Could you check a few things on this model? Use its own coordinates, in mm. A direction names the side the tool comes from. Coordinates: 2 decimals unless noted, no trailing zeros. Loops run counter-clockwise (first coordinate to the right, second up) from the corner with the lowest first, then second, coordinate; pieces in that order, holes last. Notation, with made-up numbers: (-8, 46) - (45, 46) arc R20 cw to (45, 60) - close; hole circle Ø5 at (44.25, 29). An arc over 180 degrees is marked (long way). Use CSV: the item, a comma, the result in double quotes.
Autodesk Fusion 360 part; units mm, degrees
sketch "Sketch1" plane through (0, 0, 0) normal (0, 0, 1) x (1, 0, 0)
  arc A0 (-0.5916, 85.05) -> (-0.493, 85.1333) centre (-0.5916, 85.15) ccw
  line L0 (-0.5916, 85.05) -> (-0.9084, 85.05)
  arc A1 (-1.007, 85.1333) -> (-1.5833, 84.557) centre (-1.5, 85.05) ccw
  arc A2 (0.0833, 84.557) -> (-0.493, 85.1333) centre (0, 85.05) ccw
  arc A3 (-1.007, 85.1333) -> (-0.9084, 85.05) centre (-0.9084, 85.15) ccw
  arc A4 (-1.5, 84.4584) -> (-1.5833, 84.557) centre (-1.6, 84.4584) ccw
  line L1 (-1.5, 84.4584) -> (-1.5, 0.5916)
  line L2 (0, 0.5916) -> (0, 84.4584)
  arc A5 (0.0833, 84.557) -> (0, 84.4584) centre (0.1, 84.4584) ccw
  line L3 (-1.5, 42.525) -> (0, 42.525) construction
  arc A6 (0, 0.5916) -> (0.0833, 0.493) centre (0.1, 0.5916) ccw
  arc A7 (-1.5833, 0.493) -> (-1.5, 0.5916) centre (-1.6, 0.5916) ccw
  arc A8 (-0.9084, 0) -> (-1.007, -0.0833) centre (-0.9084, -0.1) ccw
  arc A9 (-1.5833, 0.493) -> (-1.007, -0.0833) centre (-1.5, 0) ccw
  line L4 (-0.5916, 0) -> (-0.9084, 0)
  arc A10 (-0.493, -0.0833) -> (-0.5916, 0) centre (-0.5916, -0.1) ccw
  arc A11 (-0.493, -0.0833) -> (0.0833, 0.493) centre (0, 0) ccw
  line L5 (-3.5, 87.05) -> (12.65, 87.05)
  line L6 (12.65, 87.05) -> (12.65, -2)
  line L7 (12.65, -2) -> (-3.5, -2)
  line L8 (-3.5, -2) -> (-3.5, 87.05)
  line L9 (2.9334, 0) -> (2.5916, 0)
  line L10 (2, 84.4584) -> (2, 0.5916)
  arc A12 (3.6083, 84.557) -> (3.525, 84.4584) centre (3.625, 84.4584) ccw
  arc A13 (2.9334, 85.05) -> (3.032, 85.1333) centre (2.9334, 85.15) ccw
  arc A14 (1.9167, 0.493) -> (2.493, -0.0833) centre (2, 0) ccw
  arc A15 (2.493, 85.1333) -> (2.5916, 85.05) centre (2.5916, 85.15) ccw
  arc A16 (3.032, -0.0833) -> (3.6083, 0.493) centre (3.525, 0) ccw
  arc A17 (2, 84.4584) -> (1.9167, 84.557) centre (1.9, 84.4584) ccw
  arc A18 (3.525, 0.5916) -> (3.6083, 0.493) centre (3.625, 0.5916) ccw
  line L11 (2.9334, 85.05) -> (2.5916, 85.05)
  arc A19 (2.5916, 0) -> (2.493, -0.0833) centre (2.5916, -0.1) ccw
  line L12 (2, 42.525) -> (3.525, 42.525) construction
  arc A20 (2.493, 85.1333) -> (1.9167, 84.557) centre (2, 85.05) ccw
  arc A21 (3.6083, 84.557) -> (3.032, 85.1333) centre (3.525, 85.05) ccw
  arc A22 (3.032, -0.0833) -> (2.9334, 0) centre (2.9334, -0.1) ccw
  arc A23 (1.9167, 0.493) -> (2, 0.5916) centre (1.9, 0.5916) ccw
  line L13 (3.525, 0.5916) -> (3.525, 84.4584)
  arc A24 (5.4417, 0.493) -> (6.018, -0.0833) centre (5.525, 0) ccw
  line L14 (10.65, 0.5916) -> (10.65, 84.4584)
  line L15 (7.075, 0.5916) -> (7.075, 84.4584)
  line L16 (9.075, 42.525) -> (10.65, 42.525) construction
  arc A25 (9.568, 85.1333) -> (8.9917, 84.557) centre (9.075, 85.05) ccw
  line L17 (5.525, 84.4584) -> (5.525, 0.5916)
  arc A26 (6.582, -0.0833) -> (7.1583, 0.493) centre (7.075, 0) ccw
  arc A27 (10.157, -0.0833) -> (10.7333, 0.493) centre (10.65, 0) ccw
  arc A28 (6.018, 85.1333) -> (5.4417, 84.557) centre (5.525, 85.05) ccw
  line L18 (10.0584, 85.05) -> (9.6666, 85.05)
  arc A29 (8.9917, 0.493) -> (9.075, 0.5916) centre (8.975, 0.5916) ccw
  line L19 (6.4834, 0) -> (6.1166, 0)
  arc A30 (6.018, 85.1333) -> (6.1166, 85.05) centre (6.1166, 85.15) ccw
  arc A31 (9.568, 85.1333) -> (9.6666, 85.05) centre (9.6666, 85.15) ccw
  arc A32 (7.075, 0.5916) -> (7.1583, 0.493) centre (7.175, 0.5916) ccw
  line L20 (5.525, 42.525) -> (7.075, 42.525) construction
  arc A33 (6.1166, 0) -> (6.018, -0.0833) centre (6.1166, -0.1) ccw
  arc A34 (7.1583, 84.557) -> (7.075, 84.4584) centre (7.175, 84.4584) ccw
  line L21 (6.4834, 85.05) -> (6.1166, 85.05)
  arc A35 (9.075, 84.4584) -> (8.9917, 84.557) centre (8.975, 84.4584) ccw
  line L22 (9.075, 84.4584) -> (9.075, 0.5916)
  arc A36 (10.7333, 84.557) -> (10.65, 84.4584) centre (10.75, 84.4584) ccw
  arc A37 (6.582, -0.0833) -> (6.4834, 0) centre (6.4834, -0.1) ccw
  arc A38 (8.9917, 0.493) -> (9.568, -0.0833) centre (9.075, 0) ccw
  arc A39 (6.4834, 85.05) -> (6.582, 85.1333) centre (6.4834, 85.15) ccw
  arc A40 (7.1583, 84.557) -> (6.582, 85.1333) centre (7.075, 85.05) ccw
  arc A41 (9.6666, 0) -> (9.568, -0.0833) centre (9.6666, -0.1) ccw
  arc A42 (10.7333, 84.557) -> (10.157, 85.1333) centre (10.65, 85.05) ccw
  line L23 (10.0584, 0) -> (9.6666, 0)
  arc A43 (5.525, 84.4584) -> (5.4417, 84.557) centre (5.425, 84.4584) ccw
  arc A44 (10.65, 0.5916) -> (10.7333, 0.493) centre (10.75, 0.5916) ccw
  arc A45 (10.157, -0.0833) -> (10.0584, 0) centre (10.0584, -0.1) ccw
  arc A46 (5.4417, 0.493) -> (5.525, 0.5916) centre (5.425, 0.5916) ccw
  arc A47 (10.0584, 85.05) -> (10.157, 85.1333) centre (10.0584, 85.15) ccw
  arc A48 (9.568, 85.1333) -> (9.6666, 85.05) centre (9.6666, 85.15) ccw
  arc A49 (6.4834, 85.05) -> (6.582, 85.1333) centre (6.4834, 85.15) ccw
  arc A50 (10.0584, 85.05) -> (10.157, 85.1333) centre (10.0584, 85.15) ccw
  arc A51 (6.018, 85.1333) -> (5.4417, 84.557) centre (5.525, 85.05) ccw
  line L24 (10.0584, 85.05) -> (9.6666, 85.05)
  arc A52 (2.9334, 85.05) -> (3.032, 85.1333) centre (2.9334, 85.15) ccw
  arc A53 (10.7333, 84.557) -> (10.157, 85.1333) centre (10.65, 85.05) ccw
  arc A54 (6.018, 85.1333) -> (6.1166, 85.05) centre (6.1166, 85.15) ccw
  arc A55 (5.525, 84.4584) -> (5.4417, 84.557) centre (5.425, 84.4584) ccw
  arc A56 (2, 84.4584) -> (1.9167, 84.557) centre (1.9, 84.4584) ccw
  arc A57 (0.0833, 84.557) -> (0, 84.4584) centre (0.1, 84.4584) ccw
  arc A58 (10.7333, 84.557) -> (10.65, 84.4584) centre (10.75, 84.4584) ccw
  arc A59 (-1.007, 85.1333) -> (-1.5833, 84.557) centre (-1.5, 85.05) ccw
  line L25 (2.9334, 85.05) -> (2.5916, 85.05)
  arc A60 (3.6083, 84.557) -> (3.032, 85.1333) centre (3.525, 85.05) ccw
  arc A61 (-1.007, 85.1333) -> (-0.9084, 85.05) centre (-0.9084, 85.15) ccw
  arc A62 (7.1583, 84.557) -> (6.582, 85.1333) centre (7.075, 85.05) ccw
  arc A63 (2.493, 85.1333) -> (1.9167, 84.557) centre (2, 85.05) ccw
  arc A64 (9.075, 84.4584) -> (8.9917, 84.557) centre (8.975, 84.4584) ccw
  line L26 (-0.5916, 85.05) -> (-0.9084, 85.05)
  arc A65 (0.0833, 84.557) -> (-0.493, 85.1333) centre (0, 85.05) ccw
  arc A66 (-1.5, 84.4584) -> (-1.5833, 84.557) centre (-1.6, 84.4584) ccw
  arc A67 (-0.5916, 85.05) -> (-0.493, 85.1333) centre (-0.5916, 85.15) ccw
  arc A68 (7.1583, 84.557) -> (7.075, 84.4584) centre (7.175, 84.4584) ccw
  arc A69 (2.493, 85.1333) -> (2.5916, 85.05) centre (2.5916, 85.15) ccw
  line L27 (6.4834, 85.05) -> (6.1166, 85.05)
  arc A70 (3.6083, 84.557) -> (3.525, 84.4584) centre (3.625, 84.4584) ccw
  arc A71 (9.568, 85.1333) -> (8.9917, 84.557) centre (9.075, 85.05) ccw
  point P0 (-3.5, 87.05)
  point P1 (3.525, 0)
  point P2 (0.5, 87.05)
  point P3 (10.65, 0)
  point P4 (6.3, 0)
  dimension "d1" = 0.5
  dimension "d2" = 0.1
  dimension "d3" = 1.5
  dimension "d10" = 85.05
  dimension "d12" = 2
  dimension "d13" = 2
  dimension "d14" = 2
  dimension "d15" = 0.5
  dimension "d16" = 0.1
  dimension "d17" = 1.525
  dimension "d20" = 0.5
  dimension "d21" = 0.1
  dimension "d22" = 1.55
  dimension "d24" = 0.5
  dimension "d25" = 0.1
  dimension "d26" = 1.575
  dimension "d29" = 2
  dimension "d30" = 2
  dimension "d32" = 2
  dimension "d38" = 0.5
  dimension "d39" = 0.1
  dimension "d40" = 0.5
  dimension "d41" = 0.1
  dimension "d42" = 0.5
  dimension "d43" = 0.1
  dimension "d44" = 0.5
  dimension "d45" = 0.1
  dimension "d46" = 2
extrude "Extrude1" add sketch "Sketch1" along normal blind 14
sketch "Sketch2" plane through (0, 0, 0) normal (0, 0, -1) x (1, 0, 0)
  arc A0 (6.582, -85.1333) -> (7.1583, -84.557) centre (7.075, -85.05) ccw
  arc A1 (6.582, -85.1333) -> (6.4834, -85.05) centre (6.4834, -85.15) ccw
  line L0 (6.4834, -85.05) -> (6.1166, -85.05)
  arc A2 (6.1166, -85.05) -> (6.018, -85.1333) centre (6.1166, -85.15) ccw
  arc A3 (5.4417, -84.557) -> (6.018, -85.1333) centre (5.525, -85.05) ccw
  arc A4 (5.4417, -84.557) -> (5.525, -84.4584) centre (5.425, -84.4584) ccw
  line L1 (5.525, -84.4584) -> (5.525, -0.5916)
  arc A5 (5.525, -0.5916) -> (5.4417, -0.493) centre (5.425, -0.5916) ccw
  arc A6 (6.018, 0.0833) -> (5.4417, -0.493) centre (5.525, 0) ccw
  arc A7 (6.018, 0.0833) -> (6.1166, 0) centre (6.1166, 0.1) ccw
  line L2 (6.1166, 0) -> (6.4834, 0)
  arc A8 (6.4834, 0) -> (6.582, 0.0833) centre (6.4834, 0.1) ccw
  arc A9 (7.1583, -0.493) -> (6.582, 0.0833) centre (7.075, 0) ccw
  arc A10 (7.1583, -0.493) -> (7.075, -0.5916) centre (7.175, -0.5916) ccw
  line L3 (7.075, -0.5916) -> (7.075, -84.4584)
  arc A11 (7.075, -84.4584) -> (7.1583, -84.557) centre (7.175, -84.4584) ccw
  line L4 (10.0584, -85.05) -> (9.6666, -85.05)
  arc A12 (9.6666, -85.05) -> (9.568, -85.1333) centre (9.6666, -85.15) ccw
  arc A13 (8.9917, -84.557) -> (9.568, -85.1333) centre (9.075, -85.05) ccw
  arc A14 (8.9917, -84.557) -> (9.075, -84.4584) centre (8.975, -84.4584) ccw
  line L5 (9.075, -84.4584) -> (9.075, -0.5916)
  arc A15 (9.075, -0.5916) -> (8.9917, -0.493) centre (8.975, -0.5916) ccw
  arc A16 (9.568, 0.0833) -> (8.9917, -0.493) centre (9.075, 0) ccw
  arc A17 (9.568, 0.0833) -> (9.6666, 0) centre (9.6666, 0.1) ccw
  line L6 (9.6666, 0) -> (10.0584, 0)
  arc A18 (10.0584, 0) -> (10.157, 0.0833) centre (10.0584, 0.1) ccw
  arc A19 (10.7333, -0.493) -> (10.157, 0.0833) centre (10.65, 0) ccw
  arc A20 (10.7333, -0.493) -> (10.65, -0.5916) centre (10.75, -0.5916) ccw
  line L7 (10.65, -0.5916) -> (10.65, -84.4584)
  arc A21 (10.65, -84.4584) -> (10.7333, -84.557) centre (10.75, -84.4584) ccw
  arc A22 (10.157, -85.1333) -> (10.7333, -84.557) centre (10.65, -85.05) ccw
  arc A23 (10.157, -85.1333) -> (10.0584, -85.05) centre (10.0584, -85.15) ccw
  line L8 (2.9334, -85.05) -> (2.5916, -85.05)
  arc A24 (2.5916, -85.05) -> (2.493, -85.1333) centre (2.5916, -85.15) ccw
  arc A25 (1.9167, -84.557) -> (2.493, -85.1333) centre (2, -85.05) ccw
  arc A26 (1.9167, -84.557) -> (2, -84.4584) centre (1.9, -84.4584) ccw
  line L9 (2, -84.4584) -> (2, -0.5916)
  arc A27 (2, -0.5916) -> (1.9167, -0.493) centre (1.9, -0.5916) ccw
  arc A28 (2.493, 0.0833) -> (1.9167, -0.493) centre (2, 0) ccw
  arc A29 (2.493, 0.0833) -> (2.5916, 0) centre (2.5916, 0.1) ccw
  line L10 (2.5916, 0) -> (2.9334, 0)
  arc A30 (2.9334, 0) -> (3.032, 0.0833) centre (2.9334, 0.1) ccw
  arc A31 (3.6083, -0.493) -> (3.032, 0.0833) centre (3.525, 0) ccw
  arc A32 (3.6083, -0.493) -> (3.525, -0.5916) centre (3.625, -0.5916) ccw
  line L11 (3.525, -0.5916) -> (3.525, -84.4584)
  arc A33 (3.525, -84.4584) -> (3.6083, -84.557) centre (3.625, -84.4584) ccw
  arc A34 (3.032, -85.1333) -> (3.6083, -84.557) centre (3.525, -85.05) ccw
  arc A35 (3.032, -85.1333) -> (2.9334, -85.05) centre (2.9334, -85.15) ccw
  arc A36 (-1.5833, -84.557) -> (-1.007, -85.1333) centre (-1.5, -85.05) ccw
  arc A37 (-1.5833, -84.557) -> (-1.5, -84.4584) centre (-1.6, -84.4584) ccw
  line L12 (-1.5, -84.4584) -> (-1.5, -0.5916)
  arc A38 (-1.5, -0.5916) -> (-1.5833, -0.493) centre (-1.6, -0.5916) ccw
  arc A39 (-1.007, 0.0833) -> (-1.5833, -0.493) centre (-1.5, 0) ccw
  arc A40 (-1.007, 0.0833) -> (-0.9084, 0) centre (-0.9084, 0.1) ccw
  line L13 (-0.9084, 0) -> (-0.5916, 0)
  arc A41 (-0.5916, 0) -> (-0.493, 0.0833) centre (-0.5916, 0.1) ccw
  arc A42 (0.0833, -0.493) -> (-0.493, 0.0833) centre (0, 0) ccw
  arc A43 (0.0833, -0.493) -> (0, -0.5916) centre (0.1, -0.5916) ccw
  line L14 (0, -0.5916) -> (0, -84.4584)
  arc A44 (0, -84.4584) -> (0.0833, -84.557) centre (0.1, -84.4584) ccw
  arc A45 (-0.493, -85.1333) -> (0.0833, -84.557) centre (0, -85.05) ccw
  arc A46 (-0.493, -85.1333) -> (-0.5916, -85.05) centre (-0.5916, -85.15) ccw
  line L15 (-0.5916, -85.05) -> (-0.9084, -85.05)
  arc A47 (-0.9084, -85.05) -> (-1.007, -85.1333) centre (-0.9084, -85.15) ccw
  line L16 (12.65, 2) -> (-3.5, 2)
  line L17 (-3.5, 2) -> (-3.5, -87.05)
  line L18 (-3.5, -87.05) -> (12.65, -87.05)
  line L19 (12.65, -87.05) -> (12.65, 2)
  line L20 (12.65, -87.05) -> (-3.5, -87.05)
  line L21 (-3.5, -87.05) -> (-3.5, 2)
  line L22 (-3.5, 2) -> (12.65, 2)
  line L23 (12.65, 2) -> (12.65, -87.05)
extrude "Extrude2" add sketch "Sketch2" along normal blind 1 contours A0 A1 L0 A2 A3 A4 L1 A5 A6 A7 L2 A8 A9 A10 L3 A11 | L4 A12 A13 A14 L5 A15 A16 A17 L6 A18 A19 A20 L7 A21 A22 A23 | L8 A24 A25 A26 L9 A27 A28 A29 L10 A30 A31 A32 L11 A33 A34 A35 | A36 A37 L12 A38 A39 A40 L13 A41 A42 A43 L14 A44 A45 A46 L15 A47 | L16 L17 L18 L19 L20 L21 L22 L23
equation "d14 = d12"
equation "d26 = 1.55 mm + 0.025 mm"
equation "d29 = d13"
equation "d30 = d13"
equation "d32 = d13"
(1) Which directions (+Z, -Z, +X, -X, +Y, -Y) give clear straight access to the entire face, cutting with the end or side of a thin tool? Please do faces 4 (the face through (3, 42, 0)), 5 (the face through (5, -2, 6)).
Computed:
face 4,"+Z"
face 5,"+Z, -Z, +X, -X, -Y"
(2) Thinking about a two-plate mould opening in X: for faces 1 (the face through (12.65, 43, 6)), 2 (the face through (2, 43, 7)), 3 (the face through (-3.5, 42, 6)), which applies, +X half, -X half, draft (parallel to the pull), parting line (faces both ways), or undercut?
Computed:
face 1,"+X half"
face 2,"undercut"
face 3,"-X half"
(3) Will this pin go through, and if not, where does the flat tip stop? pin 1 (2 mm diameter, centred on x = 6, y = 63.5, fed in from +Z).
Computed:
pin 1,"stops at z = 14"
(4) Suppose I cut it at A-A (y = 51.5). Write out the boundary of the cut face in (x, z) (3 decimals), plus the area to 3 significant figures.
Computed:
outline,"(-3.5, -1) - (12.65, -1) - (12.65, 14) - (10.65, 14) - (10.65, 0) - (9.075, 0) - (9.075, 14) - (7.075, 14) - (7.075, 0) - (5.525, 0) - (5.525, 14) - (3.525, 14) - (3.525, 0) - (2, 0) - (2, 14) - (0, 14) - (0, 0) - (-1.5, 0) - (-1.5, 14) - (-3.5, 14) - close"
area,"156 mm²"
(5) Please list where these lines run through material, in increasing order: line 1 (X direction, y = 56.5, z = 5) (3 decimals); line 2 (Y direction, x = 10, z = 12.25); line 3 (Y direction, x = 1.75, z = 5.75).
Computed:
line 1,"x = -3.5 to -1.5, 0 to 2, 3.525 to 5.525, 7.075 to 9.075, 10.65 to 12.65"
line 2,"y = -2 to 0, 85.05 to 87.05"
line 3,"y = -2 to -0.43, 0.43 to 84.62, 85.48 to 87.05"
(6) Suppose I cut it at B-B (z = 7). State how many separate pieces and enclosed holes the cut face has, plus the area to 3 significant figures.
Computed:
separate pieces,"1"
enclosed holes,"4"
area,"906 mm²"
